Design review of the part shown in the three views and the two pictorial views. Dimensions are in mm from the part's minimum x, y and z. Coordinates: 2 decimals unless noted, no trailing zeros. Write each loop counter-clockwise with the first axis right and the second up, starting at its lowest first coordinate (ties: lowest second). Pieces come first, ordered by that corner, then holes. Notation, with made-up numbers: (1, -29) - (30, -29) arc R31 cw to (30, 7) - close; hole circle Ø6 at (-19, -22.5). An arc over 180 degrees is marked (long way). Return JSON: item names as keys, results as strings. Group by question number.
(1) For pin 1 Ø3 at (x, y) = (5, 24) entering from +Z; pin 2 Ø1 at (x, z) = (12, 79) entering from +Y; pin 3 Ø6 at (x, z) = (11, 11.5) entering from +Y, all flat-tipped, find the tip position at first contact; note any pin that passes through.
(2) To check wall thickness, follow L1, parallel to Z at x = 10.25, y = 50; L2, parallel to Z at x = 14.5, y = 50; L3, parallel to Z at x = 7.25, y = 30. State the ranges of each line that lie inside material, in increasing order. Write a range as from..to.
(3) We need section A-A on z = 50. State the section outline as (x, y) points, then the cut area to 3 significant figures.
(4) We need section B-B on x = 11.75. State the section outline as (y, z) points, then the cut area to 3 significant figures.
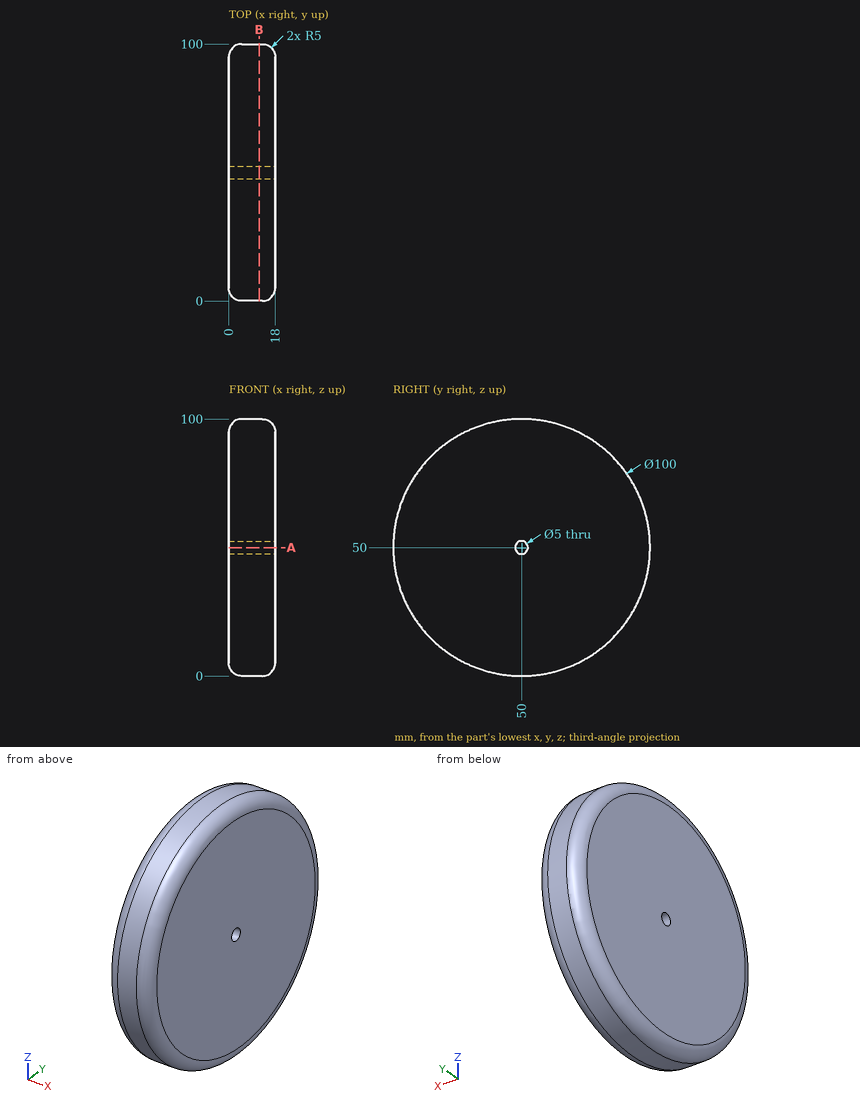
Ans:
{
 "1": {"pin 1": "z = 93.59", "pin 2": "y = 91.08", "pin 3": "y = 85.21"},
 "2": {"L1": "0..47.5, 52.5..100", "L2": "0.23..47.5, 52.5..99.77", "L3": "4.17..95.83"},
 "3": {"outline": "(0, 5) arc R5 ccw to (5, 0) - (13, 0) arc R5 ccw to (18, 5) - (18, 47.5) - (0, 47.5) - close; (0, 52.5) - (18, 52.5) - (18, 95) arc R5 ccw to (13, 100) - (5, 100) arc R5 ccw to (0, 95) - close", "area": "1,690 mm²"},
 "4": {"outline": "circle Ø100 at (50, 50); hole circle Ø5 at (50, 50)", "area": "7,830 mm²"}
}
